Autodesk Inventor part; units mm, degrees
ref_plane "YZ Plane" through (0, 0, 0) normal (1, 0, 0) x (0, 1, 0)
ref_plane "XZ Plane" through (0, 0, 0) normal (0, 1, 0) x (-1, 0, 0)
ref_plane "XY Plane" through (0, 0, 0) normal (0, 0, 1) x (1, 0, 0)
sketch "Sketch1" plane through (0, 0, 0) normal (0, 0, 1) x (1, 0, 0)
  line L0 (3.175, 0) -> (41.275, 0)
  line L1 (44.45, 3.175) -> (44.45, 22.225)
  line L2 (41.275, 25.4) -> (3.175, 25.4)
  line L3 (0, 22.225) -> (0, 3.175)
  circle A0 centre (6.35, 12.7) radius 2.0701
  circle A1 centre (31.75, 12.7) radius 2.0701
  circle A2 centre (12.7, 12.7) radius 2.0701
  line L4 (0, 12.7) -> (44.45, 12.7) construction
  circle A3 centre (38.1, 12.7) radius 2.0701
  arc A4 (3.175, 25.4) -> (0, 22.225) centre (3.175, 22.225) ccw
  arc A5 (44.45, 22.225) -> (41.275, 25.4) centre (41.275, 22.225) ccw
  arc A6 (41.275, 0) -> (44.45, 3.175) centre (41.275, 3.175) ccw
  arc A7 (0, 3.175) -> (3.175, 0) centre (3.175, 3.175) ccw
  point P0 (0, 0)
  point P1 (44.45, 25.4)
  point P2 (44.45, 0)
  point P3 (0, 25.4)
  dimension "d10" = 25.4
  dimension "d0" = 44.45
  dimension "d1" = 25.4
  dimension "d2" = 4.1402
  dimension "d3" = 6.35
  dimension "d7" = 25.4
  dimension "d12" = 6.35
  dimension "d15" = 25.4
  dimension "d20" = 3.175
extrude "Extrusion1" add sketch "Sketch1" along normal blind 3.175
properties part number "Bearing Mount Spacer 1-8 in" material "Aluminum 6061"
Geometry check sheet. Reference: the model listing, model coordinates, mm. Give positions to 0.01 mm unless a question says otherwise; leave off trailing zeros. Order: outer loops, then holes, each group sorted by start corner. A loop starts at its lowest first (then second) coordinate and runs counter-clockwise, first axis right, second up. Notation, with made-up numbers: M -3,-17.75 L 19,-17.75 A22 cw 19,12.25 Z; hole C -17.75,28.25 d10. An arc over 180 degrees is marked long. Use a Markdown table: item, result.
Item 1: Material ranges on line 1 along Y through (x, z) = (12.7, 0.75); line 2 along X through (y, z) = (14, 0.85); line 3 along Y through (x, z) = (30, 1.85), recorded low to high.
Answers follow:
| item | result |
|---|---|
| line 1 | y = 0 to 10.63, 14.77 to 25.4 |
| line 2 | x = 0 to 4.74, 7.96 to 11.09, 14.31 to 30.14, 33.36 to 36.49, 39.71 to 44.45 |
| line 3 | y = 0 to 11.59, 13.81 to 25.4 |
Item 2: Section check C-C (z = 2.05). Record the cut outline in (x, y) (3 decimals), and give its area (3 significant figures).
Answers follow:
| item | result |
|---|---|
| outline | M 0,3.175 A3.175 ccw 3.175,0 L 41.275,0 A3.175 ccw 44.45,3.175 L 44.45,22.225 A3.175 ccw 41.275,25.4 L 3.175,25.4 A3.175 ccw 0,22.225 Z; hole C 6.35,12.7 d4.14; hole C 12.7,12.7 d4.14; hole C 31.75,12.7 d4.14; hole C 38.1,12.7 d4.14 |
| area | 1,070 mm2 |
Item 3: Draft check along Y on faces 1 (the cylindrical face through (0.95, 0.91, 1.57)), 2 (the flat face through (22, 13, 3.175)), 3 (the cylindrical face through (29.68, 12.61, 1.57)), 4 (the flat face through (22, 25.4, 2)). Enter one of: +Y half, -Y half, draft (parallel to the pull), parting line (faces both ways), or undercut.
Answers follow:
| item | result |
|---|---|
| face 1 | -Y half |
| face 2 | draft |
| face 3 | undercut |
| face 4 | +Y half |
Item 4: Section check D-D (x = 12). Record the cut outline in (y, z) (3 decimals), and give its area (3 significant figures).
Answers follow:
| item | result |
|---|---|
| outline | M 0,0 L 10.752,0 L 10.752,3.175 L 0,3.175 Z; M 14.648,0 L 25.4,0 L 25.4,3.175 L 14.648,3.175 Z |
| area | 68.3 mm2 |
Item 5: Section check A-A (y = 12.7). Record the cut outline in (x, z) (3 decimals), and give its area (3 significant figures).
Answers follow:
| item | result |
|---|---|
| outline | M 0,0 L 4.28,0 L 4.28,3.175 L 0,3.175 Z; M 8.42,0 L 10.63,0 L 10.63,3.175 L 8.42,3.175 Z; M 14.77,0 L 29.68,0 L 29.68,3.175 L 14.77,3.175 Z; M 33.82,0 L 36.03,0 L 36.03,3.175 L 33.82,3.175 Z; M 40.17,0 L 44.45,0 L 44.45,3.175 L 40.17,3.175 Z |
| area | 88.5 mm2 |
Item 6: Section check B-B (x = 38.1). Record the cut outline in (y, z) (3 decimals).
Answers follow:
| item | result |
|---|---|
| outline | M 0,0 L 10.63,0 L 10.63,3.175 L 0,3.175 Z; M 14.77,0 L 25.4,0 L 25.4,3.175 L 14.77,3.175 Z |
